The model under review builds one solid part; all positions refer to its coordinate system, in mm. A direction names the side the tool comes from. Coordinates: 2 decimals unless noted, no trailing zeros. Loops run counter-clockwise (first coordinate to the right, second up) from the corner with the lowest first, then second, coordinate; pieces in that order, holes last. Notation, with made-up numbers: M 23,-20.75 L 75,-20.75 A31 cw 75,15.25 Z; hole C 7,-32 d6. An arc over 180 degrees is marked long. Return JSON: item names as keys, results as strings.
Solid Edge part; units mm, degrees
sketch "Sketch1" plane through (0, 0, 0) normal (0, -1, 0) x (1, 0, 0)
  circle A0 centre (0, 0) radius 57.5
extrude "Protrusion1" add sketch "Sketch1" against normal blind 1000
sketch "Sketch2" plane through (0, 1000, 0) normal (0, 1, 0) x (0, 0, -1)
  circle A0 centre (0, 0) radius 110
extrude "ExtrudedProtrusion_3" add sketch "Sketch2" along normal blind 1500
sketch "Sketch3" plane through (0, 0, 0) normal (0, -1, 0) x (0, 0, 1)
  circle A0 centre (0, 0) radius 50
extrude "ExtrudedCutout_2" cut sketch "Sketch3" against normal blind 2746.3549
properties material "Galvanized steel"
1. The part is to be moulded in two halves that separate along X. For faces 1 (the face through (47.1, 0, 17.3)), 2 (the face through (-15.02, 1232.5, 47.69)), 3 (the face through (-107.384, 1739.5, 23.846)), say which applies: released by +X, released by -X, zero draft, split by the parting line, or undercut.
Check values:
{"face 1": "zero draft", "face 2": "undercut", "face 3": "split by the parting line"}
2. To check wall thickness, follow line 1 (Z direction, x = 0, y = 1535.5); line 2 (X direction, y = 1206, z = -41.5). State the ranges of each line that lie inside material, in increasing order.
Check values:
{"line 1": "-110 to -50, 50 to 110", "line 2": "-101.87 to -27.89, 27.89 to 101.87"}
3. Add section D-D on y = 261. Give the boundary of the cut face in (x, z), plus the area to 3 significant figures.
Check values:
{"outline": "C 0,0 d115; hole C 0,0 d100", "area": "2,530 mm²"}
4. Machinability: for faces 4 (the face through (-12.465, 493, -56.133)), 5 (the face through (-47, 2500, 23)), which of the approach directions +Z, -Z, +X, -X, +Y, -Y give a long, thin tool a straight path to every point of the face, cutting with its end or side? Answer none if there is none.
Check values:
{"face 4": "-Y", "face 5": "+Z, -Z, +X, -X, +Y"}
5. Add section B-B on x = 0. Give the boundary of the cut face in (y, z), plus the area to 3 significant figures.
Check values:
{"outline": "M 0,-57.5 L 1000,-57.5 L 1000,-110 L 2500,-110 L 2500,-50 L 0,-50 Z; M 0,50 L 2500,50 L 2500,110 L 1000,110 L 1000,57.5 L 0,57.5 Z", "area": "195,000 mm²"}
6. Insertion check: pin 1 Ø4 at (y, z) = (444, -4) entering from -X; pin 2 Ø12 at (x, z) = (-55, 48) entering from -Y; pin 3 Ø12 at (y, z) = (298, 11) entering from -X. Each pin has a flat end and moves straight along its axis. Give the tip position at first contact, or say it passes through.
Check values:
{"pin 1": "x = -57.47", "pin 2": "y = 1000", "pin 3": "x = -57.28"}
7. Add section A-A on z = 0. Give the boundary of the cut face in (x, y), plus the area to 3 significant figures.
Check values:
{"outline": "M -110,1000 L -57.5,1000 L -57.5,0 L -50,0 L -50,2500 L -110,2500 Z; M 50,0 L 57.5,0 L 57.5,1000 L 110,1000 L 110,2500 L 50,2500 Z", "area": "195,000 mm²"}
8. Add section C-C on y = 1562. Give the boundary of the cut face in (x, z).
Check values:
{"outline": "C 0,0 d220; hole C 0,0 d100"}
